from build123d import *

# Parameters (mm, degrees)
SKETCH1_W           = 298.45
SKETCH1_H           = 25.4
BOSS_EXTRUDE1_DEPTH = 3.175
CUT_EXTRUDE1_DEPTH  = 4.175
FILLET1_R           = 2.54


with BuildPart() as part:
    # Sketch1 → Boss-Extrude1 (new body)
    with BuildSketch(Plane(origin=(0, 0, 0), x_dir=(1, 0, 0), z_dir=(0, 1, 0))):
        Rectangle(SKETCH1_W, SKETCH1_H)
    extrude(amount=BOSS_EXTRUDE1_DEPTH)

    # Sketch2 → Cut-Extrude1 (cut, through all)
    with BuildSketch(Plane(origin=(0, 3.175, 0), x_dir=(1, 0, 0), z_dir=(0, 1, 0))):
        Polygon((-142.875, -9.525), (-90.745115786, -9.525), (-142.875, 7.851628071), align=None)
        Polygon((-85.725, -7.851628071), (-85.725, 9.525), (-137.854884214, 9.525), align=None)
        Polygon((-76.2, -7.685517516), (-46.798699244, 9.525), (-76.2, 9.525), align=None)
        Polygon((-73.057550756, -9.525), (-14.254949244, -9.525), (-43.65625, 7.685517516), align=None)
        Polygon((-11.1125, -7.685517516), (-11.1125, 9.525), (-40.513800756, 9.525), align=None)
        Polygon((11.1125, -7.685517516), (40.513800756, 9.525), (11.1125, 9.525), align=None)
        Polygon((14.254949244, -9.525), (73.057550756, -9.525), (43.65625, 7.685517516), align=None)
        Polygon((76.2, -7.685517516), (76.2, 9.525), (46.798699244, 9.525), align=None)
        Polygon((85.725, -7.851628071), (137.854884214, 9.525), (85.725, 9.525), align=None)
        Polygon((90.745115786, -9.525), (142.875, -9.525), (142.875, 7.851628071), align=None)
    extrude(amount=-CUT_EXTRUDE1_DEPTH, mode=Mode.SUBTRACT)

    # Fillet1
    fillet1_edges = [part.edges().sort_by_distance(p)[0] for p in [
        (-43.65625, 1.5875, -7.685517516),
        (-14.254949244, 1.5875, 9.525),
        (-73.057550756, 1.5875, 9.525),
        (-40.513800756, 1.5875, -9.525),
        (-11.1125, 1.5875, -9.525),
        (-11.1125, 1.5875, 7.685517516),
        (-76.2, 1.5875, 7.685517516),
        (-76.2, 1.5875, -9.525),
        (-46.798699244, 1.5875, -9.525),
        (-85.725, 1.5875, 7.851628071),
        (-137.854884214, 1.5875, -9.525),
        (-85.725, 1.5875, -9.525),
        (85.725, 1.5875, 7.851628071),
        (85.725, 1.5875, -9.525),
        (137.854884214, 1.5875, -9.525),
        (46.798699244, 1.5875, -9.525),
        (76.2, 1.5875, -9.525),
        (76.2, 1.5875, 7.685517516),
        (11.1125, 1.5875, 7.685517516),
        (11.1125, 1.5875, -9.525),
        (40.513800756, 1.5875, -9.525),
        (43.65625, 1.5875, -7.685517516),
        (73.057550756, 1.5875, 9.525),
        (14.254949244, 1.5875, 9.525),
        (90.745115786, 1.5875, 9.525),
        (142.875, 1.5875, -7.851628071),
        (142.875, 1.5875, 9.525),
        (-90.745115786, 1.5875, 9.525),
        (-142.875, 1.5875, 9.525),
        (-142.875, 1.5875, -7.851628071),
    ]]
    fillet(fillet1_edges, radius=FILLET1_R)


solid = part.part
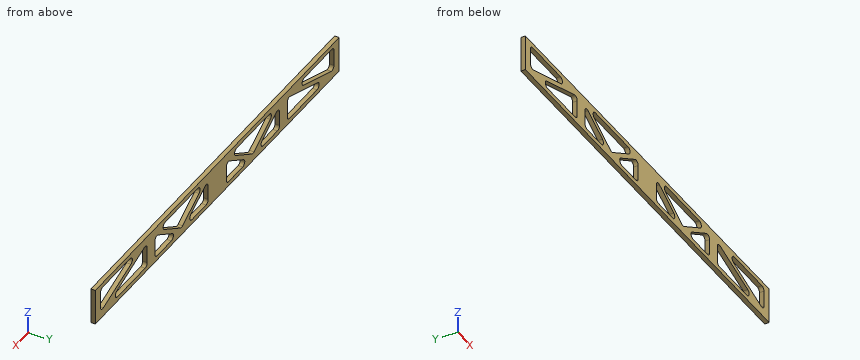
Read the model definition and answer for the solid it produces. Units are mm, in the model's axes. Give positions to 0.01 mm unless a question says otherwise; leave off trailing zeros. Write each loop counter-clockwise with the first axis right and the second up, starting at its lowest first coordinate (ties: lowest second). Pieces come first, ordered by that corner, then holes. Notation, with made-up numbers: (69.25, 63.5) -> (80.25, 63.5) arc R5 cw to (80.25, 67.5) -> close; hole circle Ø8 at (61.5, 65.25). An arc over 180 degrees is marked (long way). Answer as a JSON object with one key per item and string values. Group by question number.
1) Find section B-B (y = 0.9). Count the separate pieces of the cut face and the enclosed holes in it, and give its area (3 significant figures).
2) Consider L1, parallel to Z at x = 99.5, y = 2.25 (3 decimals); L2, parallel to Z at x = 123.5, y = 2.4 (3 decimals); L3, parallel to Z at x = -115, y = 2.9 (3 decimals). Determine where each line is inside the solid, lowest interval first. Write a range as from..to.
3) Find section A-A (x = -117). Write down the section's boundary in (y, z) (3 decimals).
Values follow:
{
 "1": {"separate pieces": "1", "enclosed holes": "10", "area": "4,030 mm2"},
 "2": {"L1": "z = -12.7..-9.525, 3.26..12.7", "L2": "z = -12.7..-9.169, -4.801..-1.393, 9.525..12.7", "L3": "z = -12.7..-9.525, -1.907..1.44, 9.525..12.7"},
 "3": {"outline": "(0, -12.7) -> (3.175, -12.7) -> (3.175, -9.525) -> (0, -9.525) -> close; (0, -2.573) -> (3.175, -2.573) -> (3.175, 0.773) -> (0, 0.773) -> close; (0, 9.525) -> (3.175, 9.525) -> (3.175, 12.7) -> (0, 12.7) -> close"}
}
